Read the model definition and answer for the solid it produces. Units are mm, in the model's axes. Face numbers are marked on the shaded views. A direction names the side the tool comes from. Coordinates: 2 decimals unless noted, no trailing zeros. Write each loop counter-clockwise with the first axis right and the second up, starting at its lowest first coordinate (ties: lowest second). Pieces come first, ordered by that corner, then holes.
1) The part is cut by section D-D (x = -16.5). Determine the outline of the cut face in (y, z).
2) The part is cut by section B-B (z = 25.5). Determine the outline of the cut face in (x, y), then the cut area to 3 significant figures.
3) Determine the mould class of the marked faces 1, 2 and 3 for opening direction Y: +Y half, -Y half, draft (parallel to the pull), parting line (faces both ways), or undercut.
4) The part is cut by section C-C (z = 30). Determine the outline of the cut face in (x, y).
5) Find the intervals of material crossed by line 1 (X direction, y = -16.1, z = 29.3); line 2 (Y direction, x = 0, z = -0.75); line 3 (Z direction, x = 20, y = -18.05), in increasing order.
6) The part is cut by section A-A (x = 0). Determine the outline of the cut face in (y, z).
7) Each of these flat-tipped pins is pushed along its axis until it touches: pin 1 Ø1.7 at (x, y) = (-11.5, 4.5) entering from +Z; pin 2 Ø10 at (y, z) = (-5.5, -1.5) entering from +X; pin 3 Ø3.5 at (x, z) = (20, 29.3) entering from -Y; pin 4 Ø10 at (y, z) = (-3, -2) entering from -X. Where does it stop, or does it pass through?
8) Which of the six approach directions +Z, -Z, +X, -X, +Y, -Y give full straight-line access (tool end or side, diameter ignored) to the marked faces 4, 5, 6, 7 and 8?
from build123d import *

# Parameters (mm, degrees)
SKETCH_1_R           = 7.5
EXTRUDE_1_DEPTH      = 6.3
CUT_EXTRUDE_1_DEPTH  = 4
SKETCH_3_R           = 2
CUT_EXTRUDE_2_DEPTH  = 41.027365639
CHAMFER_1_SIZE       = 0.5
EXTRUDE_2_DEPTH      = 28
EXTRUDE_2_DEPTH_BACK = 12.6
SKETCH_5_R           = 1.5
CUT_EXTRUDE_3_DEPTH  = 46.885618662
SKETCH_6_W           = 25
SKETCH_6_H           = 28
CUT_EXTRUDE_4_DEPTH  = 46.885618662
SKETCH_7_W           = 10
SKETCH_7_H           = 22.359066313
SKETCH_7_W_2         = 10.5
SKETCH_7_H_2         = 23.032343059
CUT_EXTRUDE_5_DEPTH  = 42.388404173
FILLET_1_R           = 3


with BuildPart() as part:
    # Sketch 1 → Extrude 1 (new, symmetric)
    with BuildSketch(Plane.XY):
        with BuildLine():
            Line((-22.5, -20), (22.5, -20))
            Line((22.5, -20), (22.5, -15))
            Line((22.5, -15), (10.956194261, 6.017624724))
            ThreePointArc((10.956194261, 6.017624724), (0, 12.5), (-10.956194261, 6.017624724))
            Line((-10.956194261, 6.017624724), (-22.5, -15))
            Line((-22.5, -15), (-22.5, -20))
        make_face()
        Circle(SKETCH_1_R, mode=Mode.SUBTRACT)
    extrude(amount=EXTRUDE_1_DEPTH, both=True)

    # Sketch 2 → Cut-Extrude 1 (cut, symmetric)
    with BuildSketch(Plane.XY):
        with BuildLine():
            Line((22.5, -15), (12.5, -15))
            Line((12.5, -15), (12.5, 0))
            ThreePointArc((12.5, 0), (12.107898832, 3.106249486), (10.956194261, 6.017624724))
            Line((10.956194261, 6.017624724), (22.5, -15))
        make_face()
        with BuildLine():
            Line((-22.5, -15), (-12.5, -15))
            Line((-12.5, -15), (-12.5, 0))
            ThreePointArc((-12.5, 0), (-12.107898832, 3.106249486), (-10.956194261, 6.017624724))
            Line((-10.956194261, 6.017624724), (-22.5, -15))
        make_face()
    extrude(amount=CUT_EXTRUDE_1_DEPTH, both=True, mode=Mode.SUBTRACT)

    # Sketch 3 → Cut-Extrude 2 (cut, through all)
    with BuildSketch(Plane.XZ.offset(20)):
        with Locations((17.5, 0)):
            Circle(SKETCH_3_R)
        with Locations(Location((-17.5, 0, 0), (0, 0, 270))):
            Circle(SKETCH_3_R)
    extrude(amount=-CUT_EXTRUDE_2_DEPTH, mode=Mode.SUBTRACT)

    # Chamfer 1
    chamfer_1_edges = [part.edges().sort_by_distance(p)[0] for p in [
        (-7.5, 0, -6.3),
        (-7.5, 0, 6.3),
    ]]
    chamfer(chamfer_1_edges, length=CHAMFER_1_SIZE)

    # Sketch 4 → Extrude 2 (add, two sides: drawn at the far end of the back side and taken through both)
    with BuildSketch(Plane.XY.offset(6.3).offset(-EXTRUDE_2_DEPTH_BACK)):
        Polygon((-22.5, -15), (-23, -15), (-23, -20), (-22.5, -20), (23, -20), (23, -15), align=None)
    extrude(amount=EXTRUDE_2_DEPTH + EXTRUDE_2_DEPTH_BACK)

    # Sketch 5 → Cut-Extrude 3 (cut, through all)
    with BuildSketch(Plane(origin=(0, 0, 0), x_dir=(1, 0, 0), z_dir=(0, 1, 0))):
        with Locations(Location((-20, -29.3, 0), (0, 0, 270))):
            Circle(SKETCH_5_R)
        with Locations((20, -29.3)):
            Circle(SKETCH_5_R)
    extrude(amount=-CUT_EXTRUDE_3_DEPTH, mode=Mode.SUBTRACT)

    # Sketch 6 → Cut-Extrude 4 (cut, through all)
    with BuildSketch(Plane(origin=(0, 0, 0), x_dir=(1, 0, 0), z_dir=(0, 1, 0))):
        with Locations((0, -20.3)):
            Rectangle(SKETCH_6_W, SKETCH_6_H)
    extrude(amount=-CUT_EXTRUDE_4_DEPTH, mode=Mode.SUBTRACT)

    # Sketch 7 → Cut-Extrude 5 (cut, through all)
    with BuildSketch(Plane.XY.offset(6.3)):
        with Locations((-17.5, -3.820466844)):
            Rectangle(SKETCH_7_W, SKETCH_7_H)
        with Locations((17.75, -3.483828471)):
            Rectangle(SKETCH_7_W_2, SKETCH_7_H_2)
    extrude(amount=-CUT_EXTRUDE_5_DEPTH, mode=Mode.SUBTRACT)

    # Fillet 1
    fillet_1_edges = [part.edges().sort_by_distance(p)[0] for p in [
        (12.5, -15, 0),
        (-12.5, -15, 0),
    ]]
    fillet(fillet_1_edges, radius=FILLET_1_R)
    fillet_1_2_edges = [part.edges().sort_by_distance(p)[0] for p in [
        (-23, -17.5, -6.3),
        (23, -17.5, -6.3),
        (-12.5, -17.5, 34.3),
        (-23, -17.5, 34.3),
        (12.5, -17.5, 34.3),
        (23, -17.5, 34.3),
    ]]
    fillet(fillet_1_2_edges, radius=FILLET_1_R)


solid = part.part
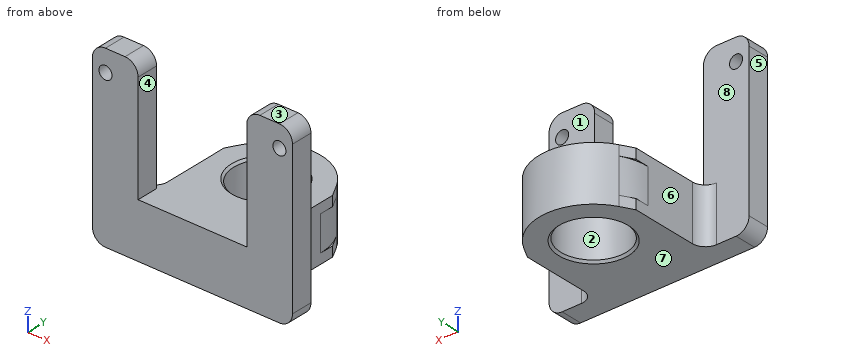
Reported:
1. outline: (-20, -6.3) - (-15, -6.3) - (-15, 34.3) - (-20, 34.3) - close
2. outline: (-23, -20) - (-12.5, -20) - (-12.5, -15) - (-23, -15) - close; (12.5, -20) - (23, -20) - (23, -15) - (12.5, -15) - close
2. area: 105 mm2
3. face 1: +Y half
3. face 2: undercut
3. face 3: draft
4. outline: (-23, -20) - (-21.33, -20) - (-21.33, -15) - (-23, -15) - close; (-18.67, -20) - (-12.5, -20) - (-12.5, -15) - (-18.67, -15) - close; (12.5, -20) - (18.67, -20) - (18.67, -15) - (12.5, -15) - close; (21.33, -20) - (23, -20) - (23, -15) - (21.33, -15) - close
5. line 1: x = -23 to -21.5, -18.5 to -12.5, 12.5 to 18.5, 21.5 to 23
5. line 2: y = -20 to -7.5, 7.5 to 12.5
5. line 3: z = -6.3 to 27.8, 30.8 to 34.3
6. outline: (-20, -6.3) - (-8, -6.3) - (-7.5, -5.8) - (-7.5, 5.8) - (-8, 6.3) - (-20, 6.3) - close; (7.5, -5.8) - (8, -6.3) - (12.5, -6.3) - (12.5, 6.3) - (8, 6.3) - (7.5, 5.8) - close
7. pin 1: stops at z = 6.3
7. pin 2: stops at x = 12.5
7. pin 3: stops at y = -20
7. pin 4: stops at x = -12.5
8. face 4: +Z, +Y, -Y
8. face 5: +Z, -Z, -X, +Y, -Y
8. face 6: +Z, -Z, -X, +Y
8. face 7: -Z, +X, -X, +Y, -Y
8. face 8: +Z, -X, +Y
